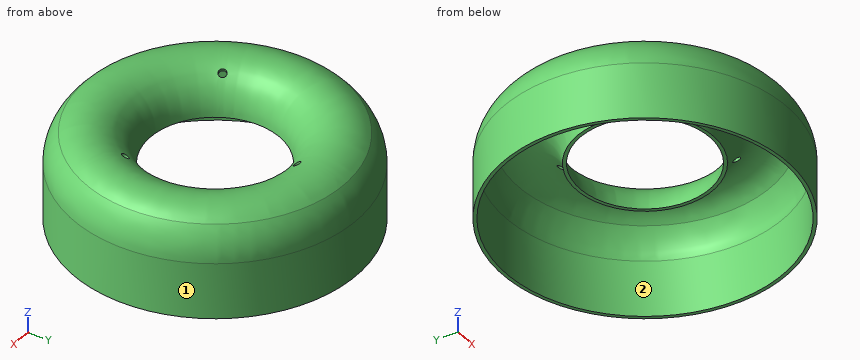
from build123d import *

# Parameters (mm, degrees)
ESQUISSE6_R                  = 1.5
ENL_V_MAT_EXTRU_5_DEPTH      = 3
R_P_TITION_CIRCULAIRE4_COUNT = 3


with BuildPart() as part:
    # Esquisse1 → Base-Révolution (revolve)
    with BuildSketch(Plane(origin=(0, 0, 0), x_dir=(0, 0, -1), z_dir=(1, 0, 0)), mode=Mode.PRIVATE) as base_r_volution_sk:
        with BuildLine():
            Line((-22.05, 25.5), (-22.05, 26.8))
            ThreePointArc((-22.05, 26.8), (-34.667475917, 34.847821439), (-32.68999151, 49.682162808))
            ThreePointArc((-32.68999151, 49.682162808), (-27.862880643, 53.19341633), (-22.05, 54.55))
            Line((-22.05, 54.55), (0, 54.55))
            Line((0, 54.55), (0, 55.85))
            Line((0, 55.85), (-21.969585692, 55.85))
            ThreePointArc((-21.969585692, 55.85), (-28.587198544, 54.596470039), (-34.190989234, 50.859938609))
            ThreePointArc((-34.190989234, 50.859938609), (-36.108183612, 34.355888829), (-22.05, 25.5))
        make_face()
    revolve(base_r_volution_sk.sketch.rotate(Axis((0, 0, 53.003727506), (0, 0, -1)), 90), axis=Axis((0, 0, 53.003727506), (0, 0, -1)))

    # Esquisse6 → Enlèv. mat.-Extru.5 (cut)
    with BuildSketch(Plane(origin=(0, -7.41473671, 12.842700706), x_dir=(-1, 0, 0), z_dir=(0, 0.49999999999999806, -0.8660254037844397))):
        with Locations(Location((0, 45.356406461, 0), (0, 0, 285.362788809))):
            Circle(ESQUISSE6_R)
    enl_v_mat_extru_5 = extrude(amount=ENL_V_MAT_EXTRU_5_DEPTH, mode=Mode.SUBTRACT)

    # Répétition circulaire4: Enlèv. mat.-Extru.5 ×3 about axis
    r_p_tition_circulaire4_axis = Axis((0, 0, 53.003727506), (0, 0, -1))
    for i in range(1, R_P_TITION_CIRCULAIRE4_COUNT):
        add(enl_v_mat_extru_5.rotate(r_p_tition_circulaire4_axis, i * 360 / R_P_TITION_CIRCULAIRE4_COUNT), mode=Mode.SUBTRACT)


solid = part.part
The model under review builds one solid part; all positions refer to its coordinate system, in mm. Face numbers are marked on the shaded views. A direction names the side the tool comes from. Give positions to 0.01 mm unless a question says otherwise; leave off trailing zeros. Order: outer loops, then holes, each group sorted by start corner. A loop starts at its lowest first (then second) coordinate and runs counter-clockwise, first axis right, second up. Notation, with made-up numbers: M 64,0 L 110,0 A14 cw 110,7 Z; hole C 34.25,79.5 d10. An arc over 180 degrees is marked long. Use one line per item in the form item = value. Start each with the question number.
Item 1: To check wall thickness, follow line 1 along Y through (x, z) = (0, 6.5); line 2 along X through (y, z) = (9, 30); line 3 along X through (y, z) = (-20, 26.5). State the ranges of each line that lie inside material, in increasing order. Write a range as from..to.
Item 2: We need section A-A on y = 0. Give the boundary of the cut face in (x, z), plus the area to 3 significant figures.
Item 3: For the marked faces 1 and 2, list the 3-axis set-ups (+Z, -Z, +X, -X, +Y, -Y) from which the entire face can be reached by the end or side of a thin tool; tool diameter is ignored.
Item 4: Insertion check: pin 1 Ø12 at (x, y) = (26, -8) entering from +Z; pin 2 Ø3 at (y, z) = (29, 6) entering from -X; pin 3 Ø6 at (x, z) = (-30, 26) entering from +Y. Each pin has a flat end and moves straight along its axis. Give the tip position at first contact, or say it passes through.
Item 5: We need section C-C on z = 8. Give the boundary of the cut face in (x, y), plus the area to 3 significant figures.
Item 6: We need section B-B on z = 30. Give the boundary of the cut face in (x, y).
Completed:
q1.line_1 = -55.85..-54.55, 54.55..55.85
q1.line_2 = -53.19..-51.21, -27.88..-26.18, 26.18..27.88, 51.21..53.19
q1.line_3 = -51.55..-49.88, -18.92..-16.85, 16.85..18.92, 49.88..51.55
q2.outline = M -55.85,0 L -54.55,0 L -54.55,22.05 A15.04 cw -49.68,32.69 A13.91 cw -26.8,22.05 L -25.5,22.05 A15.59 ccw -50.86,34.19 A16.91 ccw -55.85,21.97 Z; M 25.5,22.05 L 26.8,22.05 A13.91 cw 49.68,32.69 A15.04 cw 54.55,22.05 L 54.55,0 L 55.85,0 L 55.85,21.97 A16.91 ccw 50.86,34.19 A15.59 ccw Z
q2.area = 201 mm²
q3.face_1 = +Z, -Z
q3.face_2 = -Z
q4.pin_1 = 35.5
q4.pin_2 = -48.61
q4.pin_3 = 48.53
q5.outline = C 0,0 d111.7; hole C 0,0 d109.1
q5.area = 451 mm²
q6.outline = C 0,0 d107.88; C 0,0 d58.59; hole C 0,0 d103.99; hole C 0,0 d55.36
